For this review, use the dimensioned drawing (mm, ordinates from the lowest corner) and the shaded views. Give positions to 0.01 mm unless a question says otherwise; leave off trailing zeros. Order: outer loops, then holes, each group sorted by start corner. A loop starts at its lowest first (then second) coordinate and runs counter-clockwise, first axis right, second up.
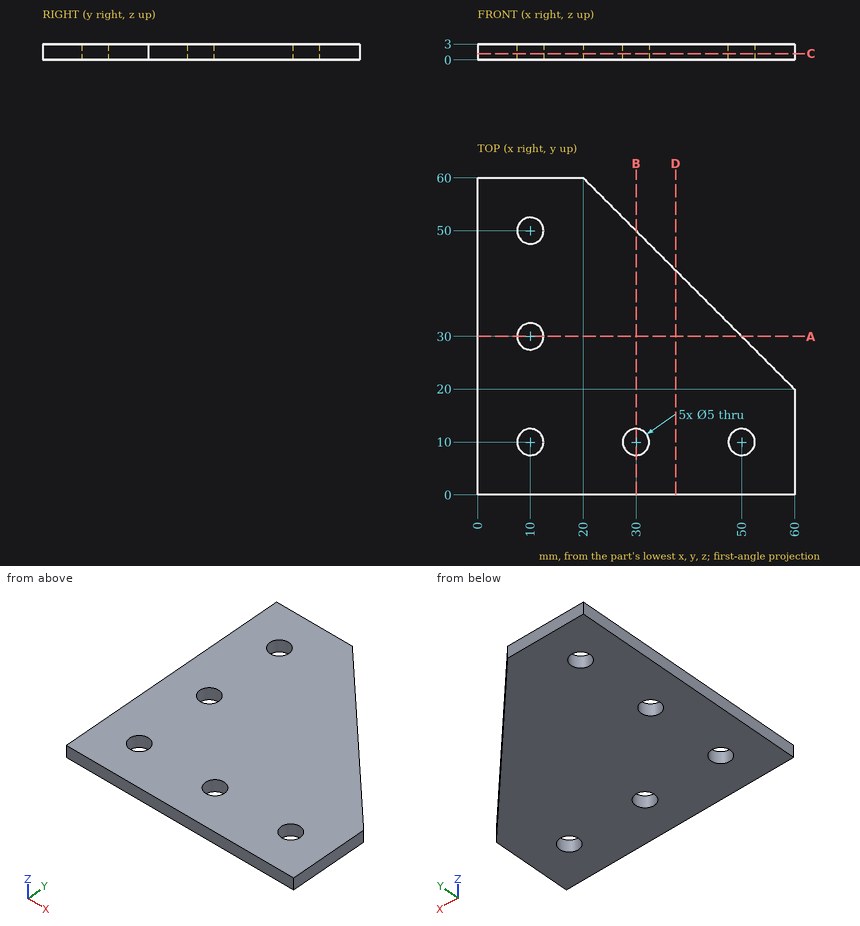
1. Take a section at A-A (y = 30). Write out the cut boundary in (x, z), and give its area (3 significant figures).
2. Take a section at C-C (z = 1.2). Write out the cut boundary in (x, y).
3. Take a section at D-D (x = 37.5). Write out the cut boundary in (y, z).
4. To check wall thickness, follow line 1 (Y direction, x = 10, z = 0.9); line 2 (Y direction, x = 48, z = 1.15); line 3 (Y direction, x = 30, z = 0.9). State the ranges of each line that lie inside material, in increasing order.
5. Insertion check: pin 1 (4.5 mm diameter, centred on x = 10, y = 50, fed in from +Z). The pin has a flat end and moves straight along its axis. Give the tip position at first contact, or say it passes through.
Answer:
1. outline: (0, 0) - (7.5, 0) - (7.5, 3) - (0, 3) - close; (12.5, 0) - (50, 0) - (50, 3) - (12.5, 3) - close
1. area: 135 mm2
2. outline: (0, 0) - (60, 0) - (60, 20) - (20, 60) - (0, 60) - close; hole circle Ø5 at (10, 10); hole circle Ø5 at (10, 30); hole circle Ø5 at (10, 50); hole circle Ø5 at (30, 10); hole circle Ø5 at (50, 10)
3. outline: (0, 0) - (42.5, 0) - (42.5, 3) - (0, 3) - close
4. line 1: y = 0 to 7.5, 12.5 to 27.5, 32.5 to 47.5, 52.5 to 60
4. line 2: y = 0 to 8.5, 11.5 to 32
4. line 3: y = 0 to 7.5, 12.5 to 50
5. pin 1: passes through
